from build123d import *

# Parameters (mm, degrees)
F0_W     = 140
F0_H     = 60
F1_DEPTH = 60
F2_R     = 10
F5_DEPTH = 10
F4_R     = 10.496877
F6_DEPTH = 69.2
F3_R     = 10
F7_DEPTH = 10
F8_R     = 5


with BuildPart() as f1:
    # F0 (on Top) → F1 (new body)
    with BuildSketch(Plane.XY):
        Rectangle(F0_W, F0_H)
    extrude(amount=F1_DEPTH)

    # F2 (on face) → F5 (join)
    with BuildSketch(Plane.XY.offset(60)):
        with Locations((-40, 0)):
            Circle(F2_R)
    extrude(amount=F5_DEPTH)

    # F4 (on face) → F6 (cut)
    with BuildSketch(Plane.XY.offset(60)):
        Circle(F4_R)
    extrude(amount=-F6_DEPTH, mode=Mode.SUBTRACT)

    # F3 (on face) → F7 (cut)
    with BuildSketch(Plane.XY.offset(60)):
        with Locations((40, 0)):
            Circle(F3_R)
    extrude(amount=-F7_DEPTH, mode=Mode.SUBTRACT)

    # F8
    f8_edges = [f1.edges().sort_by_distance(p)[0] for p in [
        (-70, 0, 60),
        (0, -30, 60),
        (70, 0, 60),
        (0, 30, 60),
    ]]
    fillet(f8_edges, radius=F8_R)


solid = f1.part
The model under review builds one solid part; all positions refer to its coordinate system, in mm. A direction names the side the tool comes from. Round coordinates to 2 decimals unless told otherwise and drop trailing zeros. Loops run counter-clockwise (first coordinate to the right, second up) from the corner with the lowest first, then second, coordinate; pieces in that order, holes last. Notation, with made-up numbers: M -32.75,-20.75 L -18.75,-20.75 A20 ccw -18.75,-10.75 Z; hole C 71,9.25 d7. An arc over 180 degrees is marked long. Answer as a JSON object with one key per item and string values.
Item 1: The part is to be moulded in two halves that separate along Y. For faces 3 (the face through (40, 0, 50)), 4 (the face through (-1, 30, 27)), 5 (the face through (30, 0, 55)), 6 (the face through (1, -29, 58)), say which applies: +Y half, -Y half, draft (parallel to the pull), parting line (faces both ways), or undercut.
Check sheet entries:
{"face 3": "undercut", "face 4": "+Y half", "face 5": "undercut", "face 6": "-Y half"}
Item 2: We need section D-D, the plane x = 27. State the section outline as (y, z) points.
Check sheet entries:
{"outline": "M -30,0 L 30,0 L 30,55 A5 ccw 25,60 L -25,60 A5 ccw -30,55 Z"}
Item 3: Clearance check with flat-ended pins moving along their axes: P1, Ø3, axis at x = -26.5, z = 57, coming from the +Y side; P2, Ø1, axis at y = 15.5, z = 59.5, coming from the -X side; P3, Ø6, axis at x = 40.5, y = 1, coming from the +Z side. State where each tip first meets the part, or that it passes through.
Check sheet entries:
{"P1": "y = 29.97", "P2": "x = -68", "P3": "z = 50"}
Item 4: We need section A-A, the plane x = 0. State the section outline as (y, z) points, and give its area (3 significant figures).
Check sheet entries:
{"outline": "M -30,0 L -10.5,0 L -10.5,60 L -25,60 A5 ccw -30,55 Z; M 10.5,0 L 30,0 L 30,55 A5 ccw 25,60 L 10.5,60 Z", "area": "2,330 mm2"}
Item 5: We need section B-B, the plane y = 0. State the section outline as (x, z) points, and give its area (3 significant figures).
Check sheet entries:
{"outline": "M -70,0 L -10.5,0 L -10.5,60 L -30,60 L -30,70 L -50,70 L -50,60 L -65,60 A5 ccw -70,55 Z; M 10.5,0 L 70,0 L 70,55 A5 ccw 65,60 L 50,60 L 50,50 L 30,50 L 30,60 L 10.5,60 Z", "area": "7,130 mm2"}
Item 6: For line 1 along Y through (x, z) = (40, 53); line 2 along Y through (x, z) = (0, 25); line 3 along Z through (x, y) = (-14, 10.5), list the stretches that pass through material, from the lowest coordinate up.
Check sheet entries:
{"line 1": "-30 to -10, 10 to 30", "line 2": "-30 to -10.5, 10.5 to 30", "line 3": "0 to 60"}
Item 7: Tool access review of faces 1 (the face through (-69, 0, 58)), 2 (the face through (-50, 0, 65)): name each direction out of +Z, -Z, +X, -X, +Y, -Y from which nothing blocks a thin tool from reaching the whole face with its end or side.
Check sheet entries:
{"face 1": "+Z, -X, +Y, -Y", "face 2": "+Z"}
Item 8: We need section C-C, the plane z = 18. State the section outline as (x, y) points, and give its area (3 significant figures).
Check sheet entries:
{"outline": "M -70,-30 L 70,-30 L 70,30 L -70,30 Z; hole C 0,0 d20.99", "area": "8,050 mm2"}
